Build history of the part. All positions in model axes, mm. Give positions to 0.01 mm unless a question says otherwise; leave off trailing zeros. Use CSV: the item, a comma, the result in double quotes. Start each with the question number.
Item 1: Wall check: line 1 along X through (y, z) = (-2.5, -292.1); line 2 along X through (y, z) = (-3.75, 190); line 3 along Z through (x, y) = (5, 3.5). Give the ranges that are in metal, low to high.
Item 2: Pin check, flat tip, straight feed: P1, Ø1, axis at x = -1, y = -1.5, coming from the -Z side. Stop position of the tip, or through.
Item 3: Band-saw the part on A-A on y = -3.25. Give the number of separate pieces and of enclosed holes in the cut face, plus the area to 3 significant figures.
from build123d import *

# Parameters (mm, degrees)
F0_W     = 25.4
F0_H     = 609.6
F1_DEPTH = 4.7625
F2_R     = 12.69999
F4_D     = 9.525


# Not quite as in the source:
# - a fillet or chamfer is up to 0.001 mm smaller than in the source, because OpenCascade refuses the exact size


with BuildPart() as f1:
    # F0 (on Front) → F1 (new body, symmetric)
    with BuildSketch(Plane.XZ):
        Rectangle(F0_W, F0_H)
    extrude(amount=F1_DEPTH, both=True)

    # F2 (radius 12.7 in the source; OpenCascade refuses exactly that, so slightly less here)
    f2_edges = [f1.edges().sort_by_distance(p)[0] for p in [
        (12.7, 0, 304.8),
        (-12.7, 0, 304.8),
        (-12.7, 0, -304.8),
        (12.7, 0, -304.8),
    ]]
    fillet(f2_edges, radius=F2_R)

    # F4 (through all)
    with Locations(Plane.XZ.offset(4.7625)):
        with Locations((0, -292.1), (0, 292.1), (0, 63.5), (0, 241.3), (0, 190.5), (0, 139.7)):
            Hole(F4_D / 2)


solid = f1.part
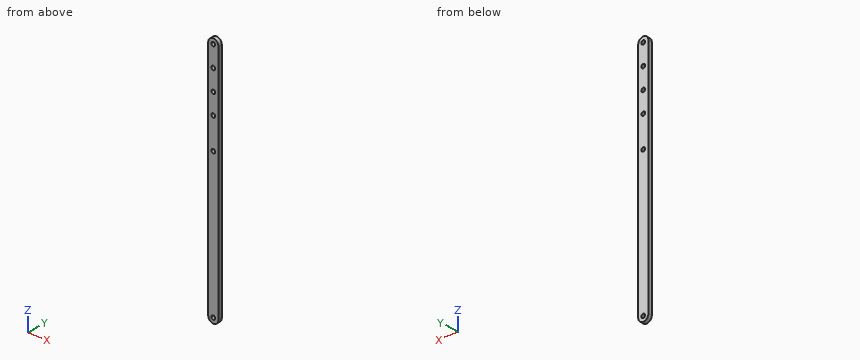
Model answer:
1,line 1,"x = -12.7 to -4.76, 4.76 to 12.7"
1,line 2,"x = -12.7 to -4.74, 4.74 to 12.7"
1,line 3,"z = -303.77 to 303.77"
2,P1,"stops at z = -304.79"
3,separate pieces,"1"
3,enclosed holes,"6"
3,area,"14,900 mm^2"
